```python
from build123d import *

# Parameters (mm, degrees)
BOX002_W     = 10
BOX002_H     = 10
BOX002_DEPTH = 8
BOX001_W     = 5
BOX001_H     = 7
BOX001_DEPTH = 10
BOX_W        = 16
BOX_H        = 16
BOX_DEPTH    = 10


with BuildPart() as cube002:
    # Box002 → Box002 (new body)
    with BuildSketch(Plane(origin=(-5, -5, 0), x_dir=(1, 0, 0), z_dir=(0, 0, 1))):
        with Locations((5, 5)):
            Rectangle(BOX002_W, BOX002_H)
    extrude(amount=BOX002_DEPTH)


with BuildPart() as cube001:
    # Box001 → Box001 (new body)
    with BuildSketch(Plane(origin=(-2.5, -3.5, 10), x_dir=(1, 0, 0), z_dir=(0, 0, 1))):
        with Locations((2.5, 3.5)):
            Rectangle(BOX001_W, BOX001_H)
    extrude(amount=BOX001_DEPTH)


with BuildPart() as cut:
    # Box → Box (new body)
    with BuildSketch(Plane(origin=(-8, -8, 0), x_dir=(1, 0, 0), z_dir=(0, 0, 1))):
        with Locations((8, 8)):
            Rectangle(BOX_W, BOX_H)
    extrude(amount=BOX_DEPTH)

    # Fusion: union Cube001
    add(cube001.part)

    # Cut: cut Cube002
    add(cube002.part, mode=Mode.SUBTRACT)


solid = cut.part
```
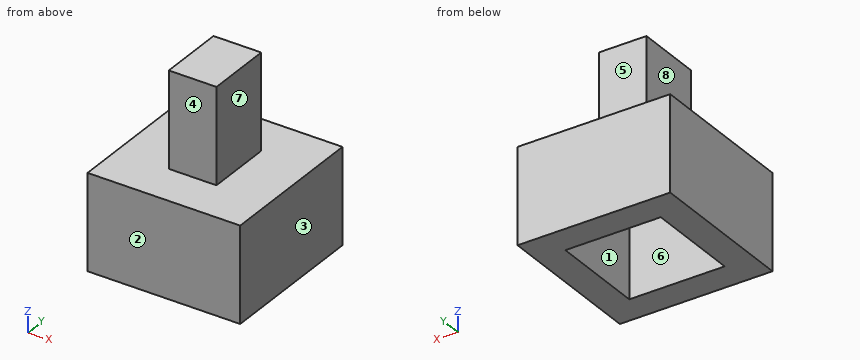
The listing builds one solid part. Answer for the finished solid, in the listing's coordinates (mm). Face numbers are marked on the shaded views. A direction names the side the tool comes from. Round coordinates to 2 decimals unless told otherwise and drop trailing zeros. Loops run counter-clockwise (first coordinate to the right, second up) from the corner with the lowest first, then second, coordinate; pieces in that order, holes last. Notation, with made-up numbers: (55, 39) - (62, 39) arc R24 cw to (62, 64) - close; hole circle Ø6 at (75, 83.25). An arc over 180 degrees is marked (long way). Use one line per item in the form item = value. Start each with the question number.
1. Consider line 1 (Y direction, x = 4, z = 2); line 2 (Z direction, x = 5.75, y = 6). Determine where each line is inside the solid, lowest interval first. Write a range as [from, to].
2. A tool of negligible diameter and unlimited length cuts with its end or side. For the marked faces 4, 5, 6, 7 and 8, from which of +Z, -Z, +X, -X, +Y, -Y can it reach the whole face along a straight path? Write none if from no direction.
3. The part is cut by section B-B on x = 1. Determine the outline of the cut face in (y, z), then the cut area to 3 significant figures.
4. For a pull along X with two mould halves and no side action, classify the marked faces 1, 2 and 3 as pulls with the +X half, pulls with the -X half, needs draft (parallel to the pull), parting line crosses it, or undercut.
5. Given pin 1 Ø4 at (x, z) = (-2.5, 17.5) entering from +Y; pin 2 Ø4 at (x, z) = (0.5, 14) entering from -Y; pin 3 Ø6 at (y, z) = (-1.5, 16) entering from +X, each flat-ended and moving along its own axis, determine where each tip first touches the part or whether it passes through.
6. The part is cut by section A-A on z = 7.25. Determine the outline of the cut face in (x, y), then the cut area to 3 significant figures.
7. The part is cut by section D-D on x = -4.5. Determine the outline of the cut face in (y, z), then the cut area to 3 significant figures.
8. The part is cut by section C-C on y = -2.5. Determine the outline of the cut face in (x, z), then the cut area to 3 significant figures.
Geometry check:
q1.line_1 = [-8, -5], [5, 8]
q1.line_2 = [0, 10]
q2.face_4 = +Z, +X, -X, -Y
q2.face_5 = +Z, +X, -X, +Y
q2.face_6 = -Z
q2.face_7 = +Z, +X, +Y, -Y
q2.face_8 = +Z, -X, +Y, -Y
q3.outline = (-8, 0) - (-5, 0) - (-5, 8) - (5, 8) - (5, 0) - (8, 0) - (8, 10) - (3.5, 10) - (3.5, 20) - (-3.5, 20) - (-3.5, 10) - (-8, 10) - close
q3.area = 150 mm^2
q4.face_1 = undercut
q4.face_2 = needs draft
q4.face_3 = pulls with the +X half
q5.pin_1 = 3.5
q5.pin_2 = -3.5
q5.pin_3 = 2.5
q6.outline = (-8, -8) - (8, -8) - (8, 8) - (-8, 8) - close; hole (-5, -5) - (5, -5) - (5, 5) - (-5, 5) - close
q6.area = 156 mm^2
q7.outline = (-8, 0) - (-5, 0) - (-5, 8) - (5, 8) - (5, 0) - (8, 0) - (8, 10) - (-8, 10) - close
q7.area = 80.0 mm^2
q8.outline = (-8, 0) - (-5, 0) - (-5, 8) - (5, 8) - (5, 0) - (8, 0) - (8, 10) - (2.5, 10) - (2.5, 20) - (-2.5, 20) - (-2.5, 10) - (-8, 10) - close
q8.area = 130 mm^2
